from build123d import *

# Parameters (mm, degrees)
SKETCH_1_R      = 50
EXTRUDE_1_DEPTH = 50
SKETCH_2_W      = 200
SKETCH_2_H      = 200
EXTRUDE_2_DEPTH = 100
FILLET_1_R      = 10


with BuildPart() as part:
    # 草图1 → 凸台-拉伸1 (new body)
    with BuildSketch(Plane.XY):
        Circle(SKETCH_1_R)
    extrude(amount=EXTRUDE_1_DEPTH)

    # 草图2 → 凸台-拉伸2 (add)
    with BuildSketch(Plane.XY.offset(50)):
        Rectangle(SKETCH_2_W, SKETCH_2_H)
    extrude(amount=EXTRUDE_2_DEPTH)

    # 圆角1
    fillet_1_edges = [part.edges().sort_by_distance(p)[0] for p in [
        (-50, 0, 0),
        (-50, 0, 50),
        (-100, 100, 100),
        (-100, -100, 100),
        (100, -100, 100),
        (100, 100, 100),
    ]]
    fillet(fillet_1_edges, radius=FILLET_1_R)


solid = part.part
Work out the finished part from the listing and answer in its coordinate system (mm). A direction names the side the tool comes from. Round coordinates to 2 decimals unless told otherwise and drop trailing zeros. Write each loop counter-clockwise with the first axis right and the second up, starting at its lowest first coordinate (ties: lowest second). Pieces come first, ordered by that corner, then holes. Notation, with made-up numbers: M 43.25,-14.5 L 48.25,-14.5 A22 cw 48.25,11.5 Z; hole C 20.25,-12.5 d1. An arc over 180 degrees is marked long. Use a Markdown table: item, result.
1) Consider line 1 (Z direction, x = 78, y = -23); line 2 (Z direction, x = 4, y = -42.5); line 3 (Y direction, x = -92, z = 102). Determine where each line is inside the solid, lowest interval first. Write a range as [from, to].
Taken from the geometry:
| item | result |
|---|---|
| line 1 | z = [50, 150] |
| line 2 | z = [0.37, 150] |
| line 3 | y = [-99.8, 99.8] |
2) Which of the six approach directions +Z, -Z, +X, -X, +Y, -Y give full straight-line access (tool end or side, diameter ignored) to faces 1 (the face through (-100, -1, 99)), 2 (the face through (-46, 46, 50))?
Taken from the geometry:
| item | result |
|---|---|
| face 1 | +Z, -Z, -X, +Y, -Y |
| face 2 | -Z |
3) The part is cut by section A-A on x = 0. Give the vertices of the cut face in (y, z), plus the area to 3 significant figures.
Taken from the geometry:
| item | result |
|---|---|
| outline | M -100,50 L -60,50 A10 cw -50,40 L -50,10 A10 ccw -40,0 L 40,0 A10 ccw 50,10 L 50,40 A10 cw 60,50 L 100,50 L 100,150 L -100,150 Z |
| area | 25,000 mm2 |
4) The part is cut by section C-C on z = 24. Give the vertices of the cut face in (x, y), plus the area to 3 significant figures.
Taken from the geometry:
| item | result |
|---|---|
| outline | C 0,0 d100 |
| area | 7,850 mm2 |
5) Flat-ended cylindrical pins translate along their axes: pin 1 (1.5 mm diameter, centred on x = 23.5, y = 70.5, fed in from -Z); pin 2 (1.5 mm diameter, centred on y = -26.5, z = 21.5, fed in from +X); pin 3 (1 mm diameter, centred on y = 4, z = 33, fed in from -X). Find the tip coordinate at first contact, or state that the pin passes through.
Taken from the geometry:
| item | result |
|---|---|
| pin 1 | stops at z = 50 |
| pin 2 | stops at x = 42.86 |
| pin 3 | stops at x = -49.88 |
